from build123d import *

# Parameters (mm, degrees)
SKETCH1_W           = 25.4
SKETCH1_H           = 12.7
BOSS_EXTRUDE1_DEPTH = 3.175
FILLET1_R           = 2.54


with BuildPart() as part:
    # Sketch1 → Boss-Extrude1 (new body)
    # profile 1 of 2: a face of its own
    with BuildSketch(Plane.XY):
        Polygon((0, 101.6), (0, 0), (12.7, 0), (12.7, 88.9), (12.7, 101.6), align=None)
        with BuildLine():
            ThreePointArc((4.445, 82.55), (6.35, 84.455), (8.255, 82.55))
            Line((8.255, 82.55), (8.255, 6.35))
            ThreePointArc((8.255, 6.35), (6.35, 4.445), (4.445, 6.35))
            Line((4.445, 6.35), (4.445, 82.55))
        make_face(mode=Mode.SUBTRACT)
    # profile 2 of 2: a face of its own
    with BuildSketch(Plane.XY):
        with Locations((25.4, 95.25)):
            Rectangle(SKETCH1_W, SKETCH1_H)
    extrude(amount=BOSS_EXTRUDE1_DEPTH)

    # Fillet1
    fillet1_edges = [part.edges().sort_by_distance(p)[0] for p in [
        (12.7, 0, 1.5875),
        (0, 0, 1.5875),
        (38.1, 101.6, 1.5875),
        (0, 101.6, 1.5875),
    ]]
    fillet(fillet1_edges, radius=FILLET1_R)


solid = part.part
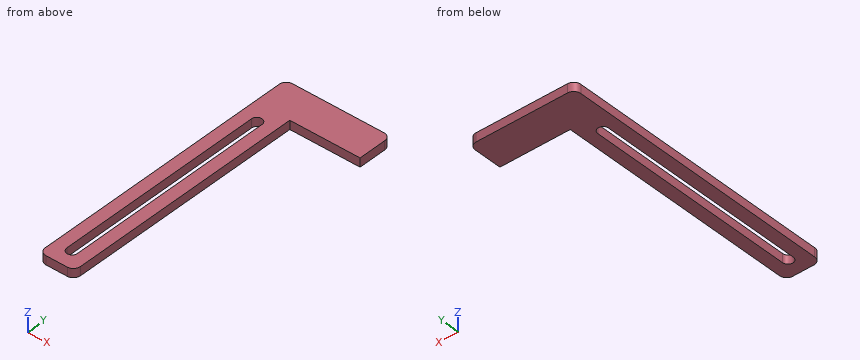
Input: part model. Units: mm. Frame: model coordinates. Give positions to 0.01 mm unless a question says otherwise; leave off trailing zeros. Order: outer loops, then holes, each group sorted by start corner. A loop starts at its lowest first (then second) coordinate and runs counter-clockwise, first axis right, second up.
Q1. Ray query, probe 1 along X at (y, z) = (43.5, 3.05) (3 decimals); probe 2 along X at (y, z) = (87, 0.4); probe 3 along Y at (x, z) = (17.5, 0.9). Return the intervals inside material, ascending.
Checked values:
probe 1: x = 0 to 4.445, 8.255 to 12.7
probe 2: x = 0 to 12.7
probe 3: y = 88.9 to 101.6
Q2. Section D-D on x = 15.5. Output: boundary loops of the cut face in (y, z) (3 decimals).
Checked values:
outline: (88.9, 0) - (101.6, 0) - (101.6, 3.175) - (88.9, 3.175) - close
Q3. Section C-C on z = 1.95. Output: boundary loops of the cut face in (x, y) (3 decimals).
Checked values:
outline: (0, 2.54) arc R2.54 ccw to (2.54, 0) - (10.16, 0) arc R2.54 ccw to (12.7, 2.54) - (12.7, 88.9) - (38.1, 88.9) - (38.1, 99.06) arc R2.54 ccw to (35.56, 101.6) - (2.54, 101.6) arc R2.54 ccw to (0, 99.06) - close; hole (4.445, 6.35) arc R1.905 ccw to (8.255, 6.35) - (8.255, 82.55) arc R1.905 ccw to (4.445, 82.55) - close
Q4. Section A-A on x = 6.35. Output: boundary loops of the cut face in (y, z) (3 decimals).
Checked values:
outline: (0, 0) - (4.445, 0) - (4.445, 3.175) - (0, 3.175) - close; (84.455, 0) - (101.6, 0) - (101.6, 3.175) - (84.455, 3.175) - close
Q5. Contact query for flat-ended pins moving along their axis: pin 1 Ø1.6 at (x, z) = (24, 1) entering from -Y; pin 2 Ø1 at (y, z) = (18.5, 2.5) entering from +X. Output: stop coordinate, or through.
Checked values:
pin 1: stops at y = 88.9
pin 2: stops at x = 12.7
Q6. Section B-B on y = 81.5. Output: boundary loops of the cut face in (x, z) (3 decimals), and give its area (3 significant figures).
Checked values:
outline: (0, 0) - (4.445, 0) - (4.445, 3.175) - (0, 3.175) - close; (8.255, 0) - (12.7, 0) - (12.7, 3.175) - (8.255, 3.175) - close
area: 28.2 mm2
